For this review, take the finished solid that the model builds, in its own axes (mm). A direction names the side the tool comes from. Round coordinates to 2 decimals unless told otherwise and drop trailing zeros. Loops run counter-clockwise (first coordinate to the right, second up) from the corner with the lowest first, then second, coordinate; pieces in that order, holes last. Notation, with made-up numbers: (35.25, 0.25) -> (67.25, 0.25) arc R24 ccw to (67.25, 39.25) -> close; hole circle Ø10 at (82, 1). An arc over 180 degrees is marked (long way). One line per question, with ' | ' between items. Start each with the question number.
1. Consider section C-C (z = 25.5). Write out the cut boundary in (x, y), and give its area (3 significant figures).
2. Draft analysis for pull direction X (two halves, no side actions). For faces 1 (the face through (44.305, -6.439, 26.436)), 2 (the face through (-11.317, -6, 6)), 3 (the face through (38.03, -6.44, 20.01)), 4 (the face through (14, 0, 23)), state which applies: pulls with the +X half, pulls with the -X half, needs draft (parallel to the pull), parting line crosses it, or undercut.
3. Consider section D-D (y = -4.25). Write out the cut boundary in (x, z), and give its area (3 significant figures).
4. Wall thickness on line 1 along X through (y, z) = (-8, 16.5); line 2 along X through (y, z) = (-6, 22.5); line 3 along Z through (x, y) = (9.5, -9.25): over which ranges is each line inside the solid? List them lowest first.
5. For faces 5 (the face through (14, -6, 21.534)), 6 (the face through (14, -6, 27.884)), list the 3-axis set-ups (+Z, -Z, +X, -X, +Y, -Y) from which the entire face can be reached by the end or side of a thin tool; tool diameter is ignored.
6. Consider section A-A (z = 9.5). Write out the cut boundary in (x, y).
7. Consider section B-B (x = 19.5). Write out the cut boundary in (y, z).
8. For pin 1 Ø4 at (x, z) = (17.93, 24.75) entering from +Y; pin 2 Ø12 at (x, z) = (-7.5, 7) entering from +Y, all flat-tipped, find the tip position at first contact; note any pin that passes through.
```python
from build123d import *

# Parameters (mm, degrees)
F0_R     = 2.499995
F1_DEPTH = 12.7
F2_R     = 5.08


with BuildPart() as f1:
    # F0 (on Front) → F1 (new body)
    with BuildSketch(Plane.XZ):
        Polygon((45.833084, 27.884173), (-17.666916, 27.884173), (-17.666916, -3.865827), (-11.316916, -3.865827), (-11.316916, 21.534173), (39.483084, 21.534173), (39.483084, -3.865827), (45.833084, -3.865827), align=None)
        with Locations((9.614785, 24.749178)):
            Circle(F0_R, mode=Mode.SUBTRACT)
        with Locations((17.933089, 24.749178)):
            Circle(F0_R, mode=Mode.SUBTRACT)
    extrude(amount=F1_DEPTH)

    # F2
    f2_edges = [f1.edges().sort_by_distance(p)[0] for p in [
        (-17.666916, -6.35, 27.884173),
        (-11.316916, -6.35, 21.534173),
        (45.833084, -6.35, 27.884173),
        (39.483084, -6.35, 21.534173),
    ]]
    fillet(f2_edges, radius=F2_R)


solid = f1.part
```
Answer block:
1) outline: (-16.89, -12.7) -> (7.23, -12.7) -> (7.23, 0) -> (-16.89, 0) -> close; (12, -12.7) -> (15.55, -12.7) -> (15.55, 0) -> (12, 0) -> close; (20.32, -12.7) -> (45.06, -12.7) -> (45.06, 0) -> (20.32, 0) -> close | area: 666 mm2
2) face 1: pulls with the +X half | face 2: undercut | face 3: undercut | face 4: needs draft
3) outline: (-17.67, -3.87) -> (-11.32, -3.87) -> (-11.32, 16.45) arc R5.08 cw to (-6.24, 21.53) -> (34.4, 21.53) arc R5.08 cw to (39.48, 16.45) -> (39.48, -3.87) -> (45.83, -3.87) -> (45.83, 22.8) arc R5.08 ccw to (40.75, 27.88) -> (-12.59, 27.88) arc R5.08 ccw to (-17.67, 22.8) -> close; hole circle Ø5 at (9.61, 24.75); hole circle Ø5 at (17.93, 24.75) | area: 687 mm2
4) line 1: x = -17.67 to -11.32, 39.48 to 45.83 | line 2: x = -17.67 to 8.52, 10.71 to 16.84, 19.02 to 45.83 | line 3: z = 21.53 to 22.25, 27.25 to 27.88
5) face 5: -Z, +Y, -Y | face 6: +Z, +X, -X, +Y, -Y
6) outline: (-17.67, -12.7) -> (-11.32, -12.7) -> (-11.32, 0) -> (-17.67, 0) -> close; (39.48, -12.7) -> (45.83, -12.7) -> (45.83, 0) -> (39.48, 0) -> close
7) outline: (-12.7, 21.53) -> (0, 21.53) -> (0, 22.8) -> (-12.7, 22.8) -> close; (-12.7, 26.7) -> (0, 26.7) -> (0, 27.88) -> (-12.7, 27.88) -> close
8) pin 1: passes through | pin 2: stops at y = 0
